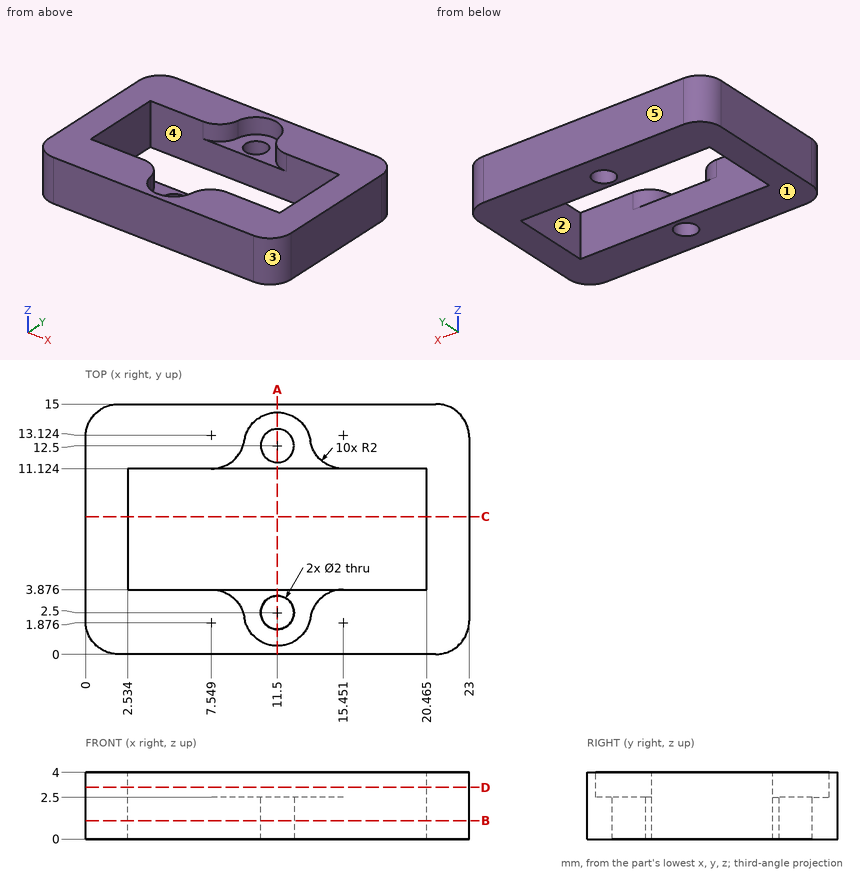
Could you check a few things on this drawing? It's one solid part, dimensions in mm from its lowest x, y, z. A direction names the side the tool comes from. Coordinates: 2 decimals unless noted, no trailing zeros. Order: outer loops, then holes, each group sorted by start corner. A loop starts at its lowest first (then second) coordinate and runs counter-clockwise, first axis right, second up. Notation, with made-up numbers: (73.5, -5) - (83.5, -5) arc R22 ccw to (83.5, 33) - close; hole circle Ø5 at (-5, 47). An arc over 180 degrees is marked (long way). Answer as a JSON object with one key per item and string values. Group by question number.
Q1. Imagine slicing it at D-D (z = 3.1). Please give me the cut outline in (x, y) (1 decimal), and give its area (3 significant figures).
Q2. Imagine slicing it at C-C (y = 8.25). Please give me the cut outline in (x, z) (1 decimal).
Q3. Imagine slicing it at B-B (z = 1.1). Please give me the cut outline in (x, y) (1 decimal).
Q4. On a 3-axis mill with a long thin cutter (end or side, diameter ignored), from which of +Z, -Z, +X, -X, +Y, -Y can I reach the whole of each face in a straight line? I mean the marked faces 1 and 2. Say none if no direction works.
Q5. Will this pin go through, and if not, where does the flat tip stop? P1, Ø2.5, axis at x = 11.5, y = 12.5, coming from the +Z side.
Q6. We'd pull the mould along Y, two halves only. Please class the marked faces 3, 4 and 5: +Y half, -Y half, draft (parallel to the pull), parting line (faces both ways), or undercut.
Q7. I need wall thicknesses on line 1 (X direction, y = 5.5, z = 2.3) (1 decimal); line 2 (Y direction, x = 6, z = 2.85) (1 decimal); line 3 (X direction, y = 2.5, z = 1.9). Which ranges of each line are inside material? Lowest first, please. Write a range as from..to.
Q8. Imagine slicing it at A-A (x = 11.5). Give the number of separate pieces and of enclosed holes in the cut face.
Determined:
{
 "1": {"outline": "(0, 2) arc R2 ccw to (2, 0) - (21, 0) arc R2 ccw to (23, 2) - (23, 13) arc R2 ccw to (21, 15) - (2, 15) arc R2 ccw to (0, 13) - close; hole (2.5, 3.9) - (7.5, 3.9) arc R2 cw to (9.5, 2.2) arc R2 ccw to (13.5, 2.2) arc R2 cw to (15.5, 3.9) - (20.5, 3.9) - (20.5, 11.1) - (15.5, 11.1) arc R2 cw to (13.5, 12.8) arc R2 ccw to (9.5, 12.8) arc R2 cw to (7.5, 11.1) - (2.5, 11.1) - close", "area": "185 mm2"},
 "2": {"outline": "(0, 0) - (2.5, 0) - (2.5, 4) - (0, 4) - close; (20.5, 0) - (23, 0) - (23, 4) - (20.5, 4) - close"},
 "3": {"outline": "(0, 2) arc R2 ccw to (2, 0) - (21, 0) arc R2 ccw to (23, 2) - (23, 13) arc R2 ccw to (21, 15) - (2, 15) arc R2 ccw to (0, 13) - close; hole (2.5, 3.9) - (20.5, 3.9) - (20.5, 11.1) - (2.5, 11.1) - close; hole circle Ø2 at (11.5, 2.5); hole circle Ø2 at (11.5, 12.5)"},
 "4": {"face 1": "-Z, +X, -X, +Y, -Y", "face 2": "+Z, -Z"},
 "5": {"P1": "stops at z = 2.5"},
 "6": {"face 3": "-Y half", "face 4": "undercut", "face 5": "+Y half"},
 "7": {"line 1": "x = 0..2.5, 20.5..23", "line 2": "y = 0..3.9, 11.1..15", "line 3": "x = 0..10.5, 12.5..23"},
 "8": {"separate pieces": "4", "enclosed holes": "0"}
}
